Build history of the part. All positions in model axes, mm. Face numbers are marked on the shaded views. A direction names the side the tool comes from. Give positions to 0.01 mm unless a question says otherwise; leave off trailing zeros. Write each loop counter-clockwise with the first axis right and the second up, starting at its lowest first coordinate (ties: lowest second). Pieces come first, ordered by that corner, then holes. Notation, with made-up numbers: (64.5, 75) -> (68.5, 75) arc R23 cw to (68.5, 92) -> close; hole circle Ø7 at (16, -39). An arc over 180 degrees is marked (long way). Write item = value, one per line. Start each with the question number.
Q1. Mould opens along X. For the marked faces 4, 5 and 6 say: pulls with the +X half, pulls with the -X half, needs draft (parallel to the pull), parting line crosses it, or undercut.
Q2. Wall check: line 1 (Z direction, x = 13.25, y = -25.3) (3 decimals); line 2 (Y direction, x = 0, z = 8.5); line 3 (Y direction, x = 16, z = 11). Give the ranges that are in metal, low to high.
Q3. Drop flat-ended pins along their axis: P1, Ø2.5, axis at x = 13.25, z = 7.5, coming from the +Y side; P2, Ø6, axis at y = 0, z = 11, coming from the -X side; P3, Ø4.5, axis at y = -13, z = 10.5, coming from the +X side; P4, Ø3, axis at x = -13.5, z = 11, coming from the +Y side. Give the stop position or say it passes through.
Q4. Saw through at A-A, the plane z = 7.5. List the corners of the cut face in (x, y) (3 decimals).
Q5. Saw through at C-C, the plane z = 11.5. List the corners of the cut face in (x, y).
Q6. Saw through at D-D, the plane x = 13.25. List the corners of the cut face in (y, z) (3 decimals), then the cut area to 4 significant figures.
Q7. Saw through at B-B, the plane x = 0. List the corners of the cut face in (y, z), then the cut area to 3 significant figures.
Q8. Tool access for the marked faces 1, 2 and 3: list every direction of +Z, -Z, +X, -X, +Y, -Y with a clear straight run to the whole face (end or side of a thin tool).
from build123d import *

# Parameters (mm, degrees)
F0_R     = 4.25
F1_DEPTH = 15
F2_R     = 2.125
F3_DEPTH = 34.751
F4_R     = 1.5


with BuildPart() as f1:
    # F0 (on Top) → F1 (new body)
    with BuildSketch(Plane.XY):
        with BuildLine():
            Line((8.25, -21.5), (8.25, 0))
            ThreePointArc((8.25, 0), (0, 8.25), (-8.25, 0))
            Line((-8.25, 0), (-8.25, -21.5))
            Line((-8.25, -21.5), (-18.25, -21.5))
            Line((-18.25, -21.5), (-18.25, -26.5))
            Line((-18.25, -26.5), (0, -26.5))
            Line((0, -26.5), (18.25, -26.5))
            Line((18.25, -26.5), (18.25, -21.5))
            Line((18.25, -21.5), (8.25, -21.5))
        make_face()
        Circle(F0_R, mode=Mode.SUBTRACT)
    extrude(amount=F1_DEPTH)

    # F2 (on face) → F3 (cut, through all)
    with BuildSketch(Plane.XZ.offset(26.5)):
        with Locations((-13.25, 7.5)):
            Circle(F2_R)
        with Locations((13.25, 7.5)):
            Circle(F2_R)
    extrude(amount=-F3_DEPTH, mode=Mode.SUBTRACT)

    # F4
    f4_edges = [f1.edges().sort_by_distance(p)[0] for p in [
        (-4.25, 0, 15),
    ]]
    fillet(f4_edges, radius=F4_R)


solid = f1.part
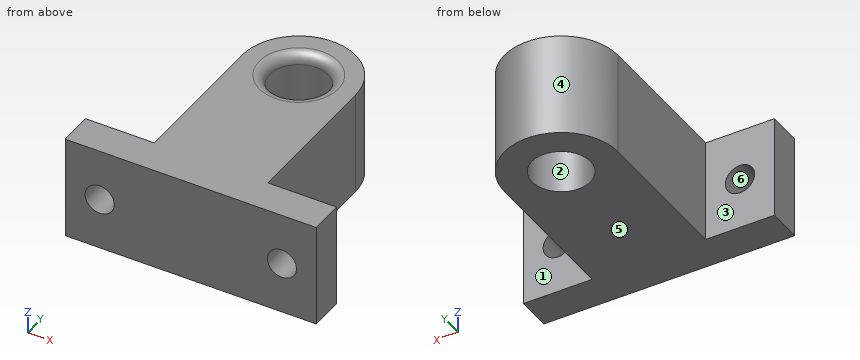
Report:
q1.face_4 = parting line crosses it
q1.face_5 = needs draft
q1.face_6 = undercut
q2.line_1 = 0 to 5.375, 9.625 to 15
q2.line_2 = -26.5 to -4.25, 4.25 to 8.25
q2.line_3 = -26.5 to -21.5
q3.P1 = through
q3.P2 = -8.25
q3.P3 = 8.25
q3.P4 = -21.5
q4.outline = (-18.25, -26.5) -> (-15.375, -26.5) -> (-15.375, -21.5) -> (-18.25, -21.5) -> close; (-11.125, -26.5) -> (11.125, -26.5) -> (11.125, -21.5) -> (8.25, -21.5) -> (8.25, 0) arc R8.25 ccw to (-8.25, 0) -> (-8.25, -21.5) -> (-11.125, -21.5) -> close; (15.375, -26.5) -> (18.25, -26.5) -> (18.25, -21.5) -> (15.375, -21.5) -> close; hole circle Ø8.5 at (0, 0)
q5.outline = (-18.25, -26.5) -> (18.25, -26.5) -> (18.25, -21.5) -> (8.25, -21.5) -> (8.25, 0) arc R8.25 ccw to (-8.25, 0) -> (-8.25, -21.5) -> (-18.25, -21.5) -> close; hole circle Ø8.5 at (0, 0)
q6.outline = (-26.5, 0) -> (-21.5, 0) -> (-21.5, 5.375) -> (-26.5, 5.375) -> close; (-26.5, 9.625) -> (-21.5, 9.625) -> (-21.5, 15) -> (-26.5, 15) -> close
q6.area = 53.75 mm2
q7.outline = (-26.5, 0) -> (-4.25, 0) -> (-4.25, 13.5) arc R1.5 ccw to (-5.75, 15) -> (-26.5, 15) -> close; (4.25, 0) -> (8.25, 0) -> (8.25, 15) -> (5.75, 15) arc R1.5 ccw to (4.25, 13.5) -> close
q7.area = 393 mm2
q8.face_1 = +Z, -Z, +X, +Y
q8.face_2 = +Z, -Z
q8.face_3 = +Z, -Z, -X, +Y
